from build123d import *

# Parameters (mm, degrees)
BOSS_EXTRU_1_DEPTH      = 2
BOSS_EXTRU_2_DEPTH      = 1.39125117
ENL_V_MAT_EXTRU_1_DEPTH = 2
BOSS_EXTRU_3_DEPTH      = 0.2
BOSS_EXTRU_3_DEPTH_BACK = 2.4
ESQUISSE4_W             = 4.9
ESQUISSE4_H             = 3.45
ESQUISSE5_W             = 2.1
ESQUISSE5_H             = 2.2
ENL_V_MAT_EXTRU_2_DEPTH = 4
ESQUISSE6_W             = 1.4
ESQUISSE6_H             = 1.55
BOSS_EXTRU_4_DEPTH      = 1.39125117
SCALE1_SCALE            = 6.5


with BuildPart() as part:
    # Esquisse1 → Boss.-Extru.1 (new body)
    with BuildSketch(Plane.XY):
        with BuildLine():
            Line((-17.95, 0), (17.95, 0))
            ThreePointArc((17.95, 0), (19.19656242, -1.520008433), (20.931194368, -0.595132491))
            ThreePointArc((20.931194368, -0.595132491), (21.146292286, 1.356483691), (20.276674314, 3.116835194))
            ThreePointArc((20.276674314, 3.116835194), (18.263317154, 3.349532273), (17.740928308, 1.39125117))
            Line((17.740928308, 1.39125117), (-17.740928308, 1.39125117))
            ThreePointArc((-17.740928308, 1.39125117), (-18.263317154, 3.349532273), (-20.276674314, 3.116835194))
            ThreePointArc((-20.276674314, 3.116835194), (-21.146292286, 1.356483691), (-20.931194368, -0.595132491))
            ThreePointArc((-20.931194368, -0.595132491), (-19.19656242, -1.520008433), (-17.95, 0))
        make_face()
        with BuildLine():
            Line((-20.534048141, 0.182330587), (-20.169386968, 2.250426868))
            ThreePointArc((-20.169386968, 2.250426868), (-18.95300824, 3.102144422), (-18.101290686, 1.885765695))
            Line((-18.101290686, 1.885765695), (-18.465951859, -0.182330587))
            ThreePointArc((-18.465951859, -0.182330587), (-19.682330587, -1.034048141), (-20.534048141, 0.182330587))
        make_face(mode=Mode.SUBTRACT)
        with BuildLine():
            Line((18.465951859, -0.182330587), (18.101290686, 1.885765695))
            ThreePointArc((18.101290686, 1.885765695), (18.95300824, 3.102144422), (20.169386968, 2.250426868))
            Line((20.169386968, 2.250426868), (20.534048141, 0.182330587))
            ThreePointArc((20.534048141, 0.182330587), (19.682330587, -1.034048141), (18.465951859, -0.182330587))
        make_face(mode=Mode.SUBTRACT)
    extrude(amount=BOSS_EXTRU_1_DEPTH)

    # Esquisse2 → Boss.-Extru.2 (add)
    with BuildSketch(Plane.XZ):
        Polygon((-16, 2), (-15.05, 2.95), (15.05, 2.95), (16, 2), align=None)
    extrude(amount=-BOSS_EXTRU_2_DEPTH)

    # Esquisse3 → Enlèv. mat.-Extru.1 (cut)
    with BuildSketch(Plane.XZ):
        Polygon((-4.5, 0), (-3.320521194, 0.55), (3.320521194, 0.55), (4.5, 0), align=None)
    extrude(amount=-ENL_V_MAT_EXTRU_1_DEPTH, mode=Mode.SUBTRACT)

    # Esquisse4 → Boss.-Extru.3 (add, two sides: drawn at the far end of the back side and taken through both)
    with BuildSketch(Plane.XY.offset(2.95).offset(-BOSS_EXTRU_3_DEPTH_BACK)):
        with Locations((0, -0.33374883)):
            Rectangle(ESQUISSE4_W, ESQUISSE4_H)
    extrude(amount=BOSS_EXTRU_3_DEPTH + BOSS_EXTRU_3_DEPTH_BACK)

    # Esquisse5 → Enlèv. mat.-Extru.2 (cut)
    with BuildSketch(Plane.XY.offset(3.15)):
        with Locations((0, -0.95874883)):
            Rectangle(ESQUISSE5_W, ESQUISSE5_H)
    extrude(amount=-ENL_V_MAT_EXTRU_2_DEPTH, mode=Mode.SUBTRACT)

    # Esquisse6 → Boss.-Extru.4 (add)
    with BuildSketch(Plane(origin=(0, 1.39125117, 0), x_dir=(1, 0, 0), z_dir=(0, 1, 0))):
        with Locations((-15.7, 0.775)):
            Rectangle(ESQUISSE6_W, ESQUISSE6_H)
        with Locations((15.7, 0.775)):
            Rectangle(ESQUISSE6_W, ESQUISSE6_H)
    extrude(amount=-BOSS_EXTRU_4_DEPTH)


with BuildPart() as part_1:
    # Scale1: scaled about (0, 0.610214787, 1.376752435)
    add(part.part.scale(SCALE1_SCALE).moved(Location((0, -3.356181328, -7.572138393))))


solid = part_1.part
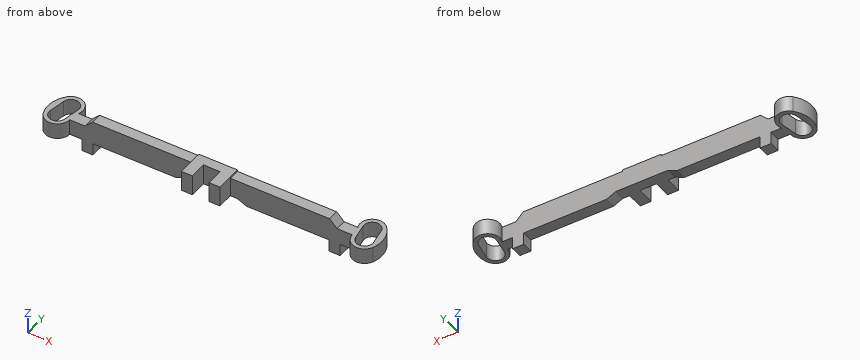
Geometry: final body of the model. Coordinates: model frame, mm. Round coordinates to 2 decimals unless told otherwise and drop trailing zeros. Loops run counter-clockwise (first coordinate to the right, second up) from the corner with the lowest first, then second, coordinate; pieces in that order, holes last. Notation, with made-up numbers: (10, 79) - (51, 79) arc R5 ccw to (51, 88) - close; hole circle Ø4 at (3, -23). An arc over 180 degrees is marked (long way). Write each question's results on one line, items separated by ' | '. Start each with the question number.
1) Cut plane C-C on x = -126.75. Return loops of the section in (y, z).
2) Cut plane B-B on y = 14. Return loops of the section in (x, z), then the cut area to 3 significant figures.
3) Line query: probe 1 along X at (y, z) = (15, 3); probe 2 along X at (y, z) = (13.5, 0); probe 3 along Z at (x, y) = (69.5, -2). Output: solid intervals per line, ascending. Write a range as [from, to].
4) Cut plane A-A on z = 3. Return loops of the section in (x, y) (3 decimals).
5) First-contact query: P1, Ø2, axis at x = -104, z = -10.5, coming from the -Y side; P2, Ø4.5, axis at y = 0, z = -14, coming from the -X side; P3, Ø17, axis at x = 128.5, y = 7, coming from the +Z side; P4, Ø8, axis at x = 35, z = -12.5, coming from the -Y side. Flat tips, straight axial feed; report the tip coordinate or a pass-through.
6) Cut plane D-D on x = -27. Return loops of the section in (y, z), then the cut area to 3 significant figures.
Verdict:
1) outline: (-13.43, -7.57) - (-10.18, -7.57) - (-10.18, 5.43) - (-13.43, 5.43) - close; (16.49, -7.57) - (19.88, -7.57) - (19.88, 5.43) - (16.49, 5.43) - close
2) outline: (-134.06, -7.57) - (-129.97, -7.57) - (-129.97, 5.43) - (-134.06, 5.43) - close; (-118.79, -7.57) - (-115.1, -7.57) - (-115.1, 5.43) - (-118.79, 5.43) - close; (115.1, -7.57) - (118.79, -7.57) - (118.79, 5.43) - (115.1, 5.43) - close; (129.97, -7.57) - (134.06, -7.57) - (134.06, 5.43) - (129.97, 5.43) - close | area: 202 mm2
3) probe 1: x = [-133.37, -129.12], [-119.64, -115.58], [115.58, 119.64], [129.12, 133.37] | probe 2: x = [-134.38, -130.29], [-118.47, -114.9], [114.9, 118.47], [130.29, 134.38] | probe 3: z = [-7.57, 11.6]
4) outline: (-136.053, -7.225) arc R10.075 ccw to (-116.675, -3.356) - (-15.925, -3.356) - (-15.925, -16.738) - (-6.825, -16.738) - (-6.825, -2.438) - (6.825, -2.438) - (6.825, -16.738) - (15.925, -16.738) - (15.925, -3.356) - (116.675, -3.356) arc R10.075 ccw to (136.053, -7.225) arc R22.75 ccw to (131.798, 16.903) arc R10.075 ccw to (115.316, 5.687) - (-115.316, 5.687) arc R10.075 ccw to (-131.798, 16.903) arc R22.75 ccw to start; hole (-133.471, -2.171) arc R6.825 ccw to (-120.029, -4.541) - (-117.658, 8.901) arc R6.825 ccw to (-131.101, 11.272) - close; hole (117.658, 8.901) - (120.029, -4.541) arc R6.825 ccw to (133.471, -2.171) - (131.101, 11.272) arc R6.825 ccw to start
5) P1: stops at y = -3.36 | P2: stops at x = -106.6 | P3: stops at z = 5.43 | P4: passes through
6) outline: (-3.36, -6.52) - (5.69, -6.52) - (5.69, 11.6) - (-3.36, 11.6) - close | area: 164 mm2
